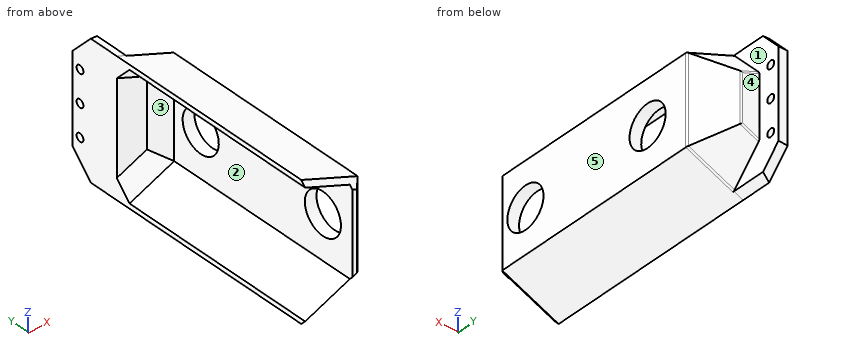
```python
from build123d import *

# Parameters (mm, degrees)
SKETCH1_W            = 30
SKETCH1_H            = 5
BOSS_EXTRUDE1_DEPTH  = 19.3
SKETCH2_W            = 40
SKETCH2_H            = 10
BOSS_EXTRUDE2_DEPTH  = 3.175
SKETCH3_W            = 4
SKETCH3_H            = 30
BOSS_EXTRUDE3_DEPTH  = 75
CUT_EXTRUDE1_REACH   = 84.48
SKETCH4_R            = 7.1
BOSS_EXTRUDE7_DEPTH  = 5
BOSS_EXTRUDE8_DEPTH  = 5
CHAMFER1_SIZE        = 5
BOSS_EXTRUDE9_DEPTH  = 75
BOSS_EXTRUDE10_DEPTH = 5
CHAMFER2_SIZE        = 5
CHAMFER3_SIZE        = 10
BOSS_EXTRUDE15_DEPTH = 3.175
CUT_EXTRUDE2_DEPTH   = 81.759021382
FILLET6_R            = 1
FILLET7_R            = 1
CHAMFER6_SIZE        = 2.5
SKETCH16_R           = 1.35
CUT_EXTRUDE3_DEPTH   = 83.406281069


with BuildPart() as part:
    # Sketch1 → Boss-Extrude1 (new body)
    with BuildSketch(Plane(origin=(0, 0, 0), x_dir=(0, 0, -1), z_dir=(1, 0, 0))):
        Rectangle(SKETCH1_W, SKETCH1_H)
    extrude(amount=BOSS_EXTRUDE1_DEPTH)

    # Sketch2 → Boss-Extrude2 (add)
    with BuildSketch(Plane.ZY):
        with Locations((0.597390222, 2.5)):
            Rectangle(SKETCH2_W, SKETCH2_H)
    extrude(amount=-BOSS_EXTRUDE2_DEPTH)

    # Sketch3 → Boss-Extrude3 (add)
    with BuildSketch(Plane.XZ.offset(2.5)):
        with Locations((17.3, 0)):
            Rectangle(SKETCH3_W, SKETCH3_H)
    extrude(amount=BOSS_EXTRUDE3_DEPTH)

    # Sketch4 → Cut-Extrude1 (cut, up to next)
    with BuildSketch(Plane(origin=(19.3, 0, 0), x_dir=(0, 0, -1), z_dir=(1, 0, 0)), mode=Mode.PRIVATE) as cut_extrude1_sk1:
        with Locations((2.035e-06, -17.9)):
            Circle(SKETCH4_R)
    cut_extrude1_tool1 = extrude(cut_extrude1_sk1.sketch, amount=-CUT_EXTRUDE1_REACH, mode=Mode.PRIVATE) & part.part
    # Sketch4 → Cut-Extrude1 (cut, up to next)
    with BuildSketch(Plane(origin=(19.3, 0, 0), x_dir=(0, 0, -1), z_dir=(1, 0, 0)), mode=Mode.PRIVATE) as cut_extrude1_sk2:
        with Locations((-1.3e-07, -65.9)):
            Circle(SKETCH4_R)
    cut_extrude1_tool2 = extrude(cut_extrude1_sk2.sketch, amount=-CUT_EXTRUDE1_REACH, mode=Mode.PRIVATE) & part.part
    add(cut_extrude1_tool1.solids().sort_by_distance((19.3, -17.9, -2e-06))[0], mode=Mode.SUBTRACT)
    add(cut_extrude1_tool2.solids().sort_by_distance((19.3, -65.9, 0))[0], mode=Mode.SUBTRACT)

    # Sketch10 → Boss-Extrude7 (add)
    with BuildSketch(Plane(origin=(0, 2.5, 0), x_dir=(1, 0, 0), z_dir=(0, 1, 0))):
        Polygon((3.175, 19.402609778), (0, 19.402609778), (0, 22.902609778), (19.3, 15), (3.175, 15), align=None)
    boss_extrude7 = extrude(amount=-BOSS_EXTRUDE7_DEPTH)

    # Sketch11 → Boss-Extrude8 (add)
    with BuildSketch(Plane(origin=(0, 2.5, 0), x_dir=(1, 0, 0), z_dir=(0, 1, 0))):
        Polygon((0, 19.402609778), (0, 22.902609778), (3.175, 21.60256905), (3.175, 19.402609778), align=None)
    boss_extrude8 = extrude(amount=BOSS_EXTRUDE8_DEPTH)

    # Mirror2: Boss-Extrude7, Boss-Extrude8 across plane
    add(boss_extrude7.mirror(Plane(origin=(0, 0, 0), x_dir=(1, 0, 0), z_dir=(0, 0, -1))))
    add(boss_extrude8.mirror(Plane(origin=(0, 0, 0), x_dir=(1, 0, 0), z_dir=(0, 0, -1))))

    # Chamfer1
    chamfer1_edges = [part.edges().sort_by_distance(p)[0] for p in [
        (3.175, 2.5, 0),
    ]]
    chamfer(chamfer1_edges, length=CHAMFER1_SIZE - 0.0001)  # a hair under: the kernel refuses the full size

    # Sketch12 → Boss-Extrude9 (add)
    with BuildSketch(Plane.XZ.offset(2.5)):
        Polygon((0, -22.902609778), (19.3, -15), (15.3, -15), (0, -21.264763192), align=None)
        Polygon((0, 22.902609778), (19.3, 15), (15.3, 15), (0, 21.264763192), align=None)
    extrude(amount=BOSS_EXTRUDE9_DEPTH)

    # Sketch13 → Boss-Extrude10 (add)
    with BuildSketch(Plane(origin=(0, 2.5, 0), x_dir=(1, 0, 0), z_dir=(0, 1, 0))):
        Polygon((3.175, 21.60256905), (3.175, -21.60256905), (19.3, -15), (19.3, 15), align=None)
    extrude(amount=BOSS_EXTRUDE10_DEPTH)

    # Chamfer2
    chamfer2_edges = [part.edges().sort_by_distance(p)[0] for p in [
        (7.65, -2.5, -18.132381596),
        (7.65, -2.5, 18.132381596),
        (15.3, -2.5, 0),
    ]]
    chamfer(chamfer2_edges, length=CHAMFER2_SIZE)

    # Chamfer3
    chamfer3_edges = [part.edges().sort_by_distance(p)[0] for p in [
        (9.65, 7.5, 18.951304889),
        (19.3, 7.5, 0),
        (9.65, 7.5, -18.951304889),
    ]]
    chamfer(chamfer3_edges, length=CHAMFER3_SIZE)

    # Sketch14 → Boss-Extrude15 (add)
    with BuildSketch(Plane.ZY):
        Polygon((-22.902609778, -2.5), (-22.902609778, 7.718772797), (-15.034642071, 15), (15.034642071, 15), (22.902609778, 7.718772797), (22.902609778, -2.5), align=None)
    extrude(amount=-BOSS_EXTRUDE15_DEPTH)

    # Sketch15 → Cut-Extrude2 (cut, through all)
    with BuildSketch(Plane.XZ.offset(2.5)):
        Polygon((3.175, 22.902609778), (0, 22.902609778), (3.175, 21.60256905), align=None)
        Polygon((3.175, -22.902609778), (3.175, -21.60256905), (0, -22.902609778), align=None)
    extrude(amount=-CUT_EXTRUDE2_DEPTH, mode=Mode.SUBTRACT)

    # Fillet6
    fillet6_edges = [part.edges().sort_by_distance(p)[0] for p in [
        (9.3, 7.5, 0),
        (6.2375, 7.5, -9.542766367),
        (6.2375, 7.5, 9.542766367),
    ]]
    fillet(fillet6_edges, radius=FILLET6_R)

    # Fillet7
    fillet7_edges = [part.edges().sort_by_distance(p)[0] for p in [
        (11.2375, -2.5, 18.301284525),
        (19.3, -2.5, 0),
        (11.2375, -2.5, -18.301284525),
    ]]
    fillet(fillet7_edges, radius=FILLET7_R)

    # Chamfer6
    chamfer6_edges = [part.edges().sort_by_distance(p)[0] for p in [
        (9.65, -77.5, -18.951304889),
        (19.3, -77.5, 0),
        (9.65, -77.5, 18.951304889),
    ]]
    chamfer(chamfer6_edges, length=CHAMFER6_SIZE)

    # Sketch16 → Cut-Extrude3 (cut, through all)
    with BuildSketch(Plane(origin=(3.175, 0, 0), x_dir=(0, 0, -1), z_dir=(1, 0, 0))):
        with Locations((0, 11.960932583)):
            Circle(SKETCH16_R)
        with Locations((-10.818605561, 11.960932583)):
            Circle(SKETCH16_R)
        with Locations((10.818605561, 11.960932583)):
            Circle(SKETCH16_R)
    extrude(amount=-CUT_EXTRUDE3_DEPTH, mode=Mode.SUBTRACT)


solid = part.part
```
Could you check a few things on this model? Use its own coordinates, in mm. Face numbers are marked on the shaded views. A direction names the side the tool comes from. Round coordinates to 2 decimals unless told otherwise and drop trailing zeros. Loops run counter-clockwise (first coordinate to the right, second up) from the corner with the lowest first, then second, coordinate; pieces in that order, holes last. Notation, with made-up numbers: M -0.5,59.5 L 36.5,59.5 A22 ccw 36.5,69.5 Z; hole C 83,-34.5 d9. An arc over 180 degrees is marked long. Answer as CSV lines item,"result".
1) If I drill on probe 1 along Y at (x, z) = (18, -2); probe 2 along Y at (x, z) = (1.1, 0); probe 3 along X at (y, z) = (-46.5, -10), over which ranges is the centre line in solid material (lowest first)?
From the geometry:
probe 1,"-76.3 to -72.71, -59.09 to -24.71, -11.09 to -1.2"
probe 2,"-2.5 to 10.61, 13.31 to 15"
probe 3,"15.3 to 19.3"
2) For pin 1 Ø15 at (y, z) = (-39, -2.5) entering from -X; pin 2 Ø3 at (x, y) = (8, -64) entering from +Z; pin 3 Ø3 at (x, z) = (2.5, -0.5) entering from -Y; pin 4 Ø8.5 at (y, z) = (-17.9, 0) entering from +X, each with a flat end and sliding along its axis, tell me the tip position at first contact or that it passes through.
From the geometry:
pin 1,"x = 15.3"
pin 2,"z = 20.24"
pin 3,"y = -2.5"
pin 4,"through"
3) Imagine slicing it at B-B on y = -17.9. List the corners of the cut face in (x, z) for me.
From the geometry:
outline,"M 0,-22.9 L 19.3,-15 L 19.3,-7.1 L 15.3,-7.1 L 15.3,-15 L 0,-21.26 Z; M 0,21.26 L 15.3,15 L 15.3,7.1 L 19.3,7.1 L 19.3,15 L 0,22.9 Z"
4) Imagine slicing it at C-C on y = -63.5. List the corners of the cut face in (x, z) for me, and give its area (3 significant figures).
From the geometry:
outline,"M 0,-22.9 L 19.3,-15 L 19.3,-6.68 L 15.3,-6.68 L 15.3,-15 L 0,-21.26 Z; M 0,21.26 L 15.3,15 L 15.3,6.68 L 19.3,6.68 L 19.3,15 L 0,22.9 Z"
area,"123 mm^2"
5) Which directions (+Z, -Z, +X, -X, +Y, -Y) give clear straight access to the entire face, cutting with the end or side of a thin tool? Please do the marked faces 3, 4 and 5.
From the geometry:
face 3,"-X, -Y"
face 4,"+Z, -Z, +X, +Y"
face 5,"+Z, -Z, +X, +Y, -Y"
6) Imagine slicing it at A-A on z = 0. List the corners of the cut face in (x, y) for me (3 decimals), and give its area (3 significant figures).
From the geometry:
outline,"M 0,-2.5 L 10.3,-2.5 L 15.3,-7.5 L 15.3,-10.8 L 19.3,-10.8 L 19.3,-2.914 A1 ccw 19.007,-2.207 L 9.593,7.207 A1 ccw 8.886,7.5 L 3.175,7.5 L 3.175,10.611 L 0,10.611 Z; M 0,13.311 L 3.175,13.311 L 3.175,15 L 0,15 Z; M 15.3,-77.5 L 16.8,-77.5 L 19.3,-75 L 19.3,-73 L 15.3,-73 Z; M 15.3,-58.8 L 19.3,-58.8 L 19.3,-25 L 15.3,-25 Z"
area,"354 mm^2"
7) We'd pull the mould along Z, two halves only. Please class the marked faces 1 and 2: released by +Z, released by -Z, zero draft, split by the parting line, or undercut.
From the geometry:
face 1,"zero draft"
face 2,"undercut"
